For this review, use the dimensioned drawing (mm, ordinates from the lowest corner) and the shaded views. Round coordinates to 2 decimals unless told otherwise and drop trailing zeros. Loops run counter-clockwise (first coordinate to the right, second up) from the corner with the lowest first, then second, coordinate; pieces in that order, holes last. Notation, with made-up numbers: M -8,68 L 49,68 A34 cw 49,102 Z; hole C -40,-18.75 d5. An arc over 180 degrees is marked long. One line per item, written item: value. Start each with the question number.
Item 1: We need section C-C (z = 33.5). Write out the cut boundary in (x, y).
Item 2: We need section D-D (z = 11). Write out the cut boundary in (x, y), then the cut area to 3 significant figures.
Item 3: Mouldability with a two-part tool opening along Y and no side actions: class the marked faces 1, 2, 3 and 4 as released by +Y, released by -Y, zero draft, split by the parting line, or undercut.
Item 4: For line 1 along Y through (x, z) = (28, 41); line 2 along X through (y, z) = (13, 21.5) (1 decimal); line 3 along Y through (x, z) = (39.5, 41.5) (1 decimal), list the stretches that pass through material, from the lowest coordinate up.
Item 5: Clearance check with flat-ended pins moving along their axes: pin 1 (12 mm diameter, centred on x = 26, z = 5.5, fed in from -Y); pin 2 (8 mm diameter, centred on x = 29.5, z = 39, fed in from -Y); pin 3 (2 mm diameter, centred on y = 20.5, z = 15.5, fed in from -X); pin 4 (5 mm diameter, centred on x = 43.5, y = 46.5, fed in from -Z). State where each tip first meets the part, or that it passes through.
Item 6: We need section A-A (y = 28). Write out the cut boundary in (x, z).
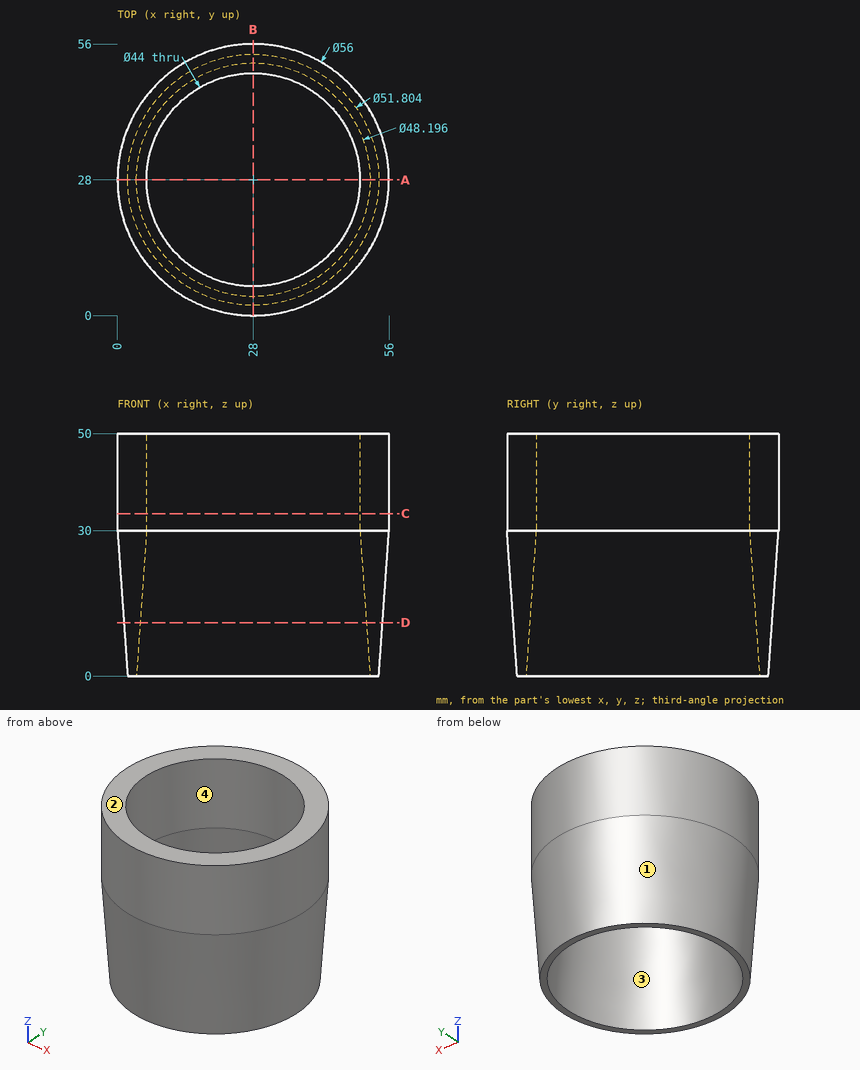
A:
1. outline: C 28,28 d56; hole C 28,28 d44
2. outline: C 28,28 d53.34; hole C 28,28 d46.66
2. area: 525 mm2
3. face 1: split by the parting line
3. face 2: zero draft
3. face 3: undercut
3. face 4: undercut
4. line 1: 0 to 6, 50 to 56
4. line 2: 5.1 to 11.1, 44.9 to 50.9
4. line 3: 2.5 to 9.2, 46.8 to 53.5
5. pin 1: y = 1.31
5. pin 2: y = 0
5. pin 3: x = 1.8
5. pin 4: z = 0
6. outline: M 0,30 L 2.1,0 L 3.9,0 L 6,30 L 6,50 L 0,50 Z; M 50,30 L 52.1,0 L 53.9,0 L 56,30 L 56,50 L 50,50 Z
